Part model, mm, in its own coordinate system. Face numbers are marked on the shaded views. Coordinates: 2 decimals unless noted, no trailing zeros. Write each loop counter-clockwise with the first axis right and the second up, starting at its lowest first coordinate (ties: lowest second). Pieces come first, ordered by that corner, then holes. Notation, with made-up numbers: M 0,-28.5 L 38,-28.5 A9 cw 38,-16.5 Z; hole C -13,46.5 d5. An arc over 180 degrees is marked long. Use a Markdown table: item, result. Add a question column.
Q1. Pin check, flat tips, straight feed: pin 1 Ø1.5 at (y, z) = (65.5, 5.5) entering from -X; pin 2 Ø4 at (x, y) = (-0.5, 16.5) entering from +Z; pin 3 Ø6 at (y, z) = (65, -6) entering from +X. Stop position of each tip, or through.
Q2. Slice it at A-A on y = 31.5. Write the cut outline in (x, z), then the cut area to 3 significant figures.
Q3. Mould opens along Z. For the marked faces 1, 2, 3 and 4 say: released by +Z, released by -Z, zero draft, split by the parting line, or undercut.
Q4. Wall check: L1, parallel to Y at x = -8, z = -6.5; L2, parallel to X at y = 91, z = 0.5; L3, parallel to Z at x = -4.75, y = 15. Give the ranges that are in metal, low to high. Write a range as from..to.
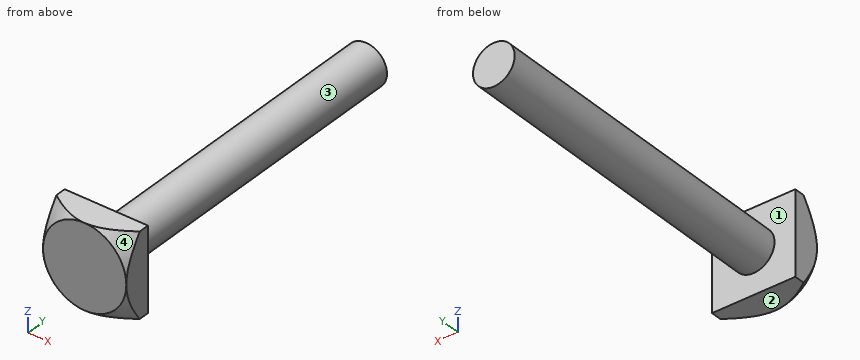
from build123d import *

# Parameters (mm, degrees)
SKETCH1_R           = 6
BOSS_EXTRUDE1_DEPTH = 96
SKETCH11_W          = 24
SKETCH11_H          = 24
BOSS_EXTRUDE5_DEPTH = 8
SKETCH12_OUTSIDE_W  = 63.88
SKETCH12_OUTSIDE_H  = 63.88
SKETCH12_OUTSIDE_R  = 12
CUT_EXTRUDE3_DEPTH  = 8
CUT_EXTRUDE3_TAPER  = 45


with BuildPart() as part:
    # Sketch1 → Boss-Extrude1 (new body)
    with BuildSketch(Plane(origin=(0, 0, 0), x_dir=(1, 0, 0), z_dir=(0, 1, 0))):
        Circle(SKETCH1_R)
    extrude(amount=BOSS_EXTRUDE1_DEPTH)

    # Sketch11 → Boss-Extrude5 (add)
    with BuildSketch(Plane.XZ):
        Rectangle(SKETCH11_W, SKETCH11_H)
    extrude(amount=BOSS_EXTRUDE5_DEPTH)

    # Sketch12 outside → Cut-Extrude3 (cut)
    with BuildSketch(Plane(origin=(0, -8, 0), x_dir=(-1, 0, 0), z_dir=(0, -1, 0))):
        Rectangle(SKETCH12_OUTSIDE_W, SKETCH12_OUTSIDE_H)
        Circle(SKETCH12_OUTSIDE_R, mode=Mode.SUBTRACT)
    extrude(amount=-CUT_EXTRUDE3_DEPTH, taper=CUT_EXTRUDE3_TAPER, mode=Mode.SUBTRACT)


solid = part.part
Recorded:
| question | item | result |
|---|---|---|
| 1 | pin 1 | x = -3.67 |
| 1 | pin 2 | z = 6 |
| 1 | pin 3 | x = 5.2 |
| 2 | outline | C 0,0 d12 |
| 2 | area | 113 mm² |
| 3 | face 1 | zero draft |
| 3 | face 2 | released by -Z |
| 3 | face 3 | split by the parting line |
| 3 | face 4 | released by +Z |
| 4 | L1 | -8..0 |
| 4 | L2 | -5.98..5.98 |
| 4 | L3 | -3.67..3.67 |
